Could you check a few things on this model? Use its own coordinates, in mm. A direction names the side the tool comes from. Coordinates: 2 decimals unless noted, no trailing zeros. Write each loop counter-clockwise with the first axis right and the second up, starting at its lowest first coordinate (ties: lowest second). Pieces come first, ordered by that corner, then holes. Notation, with made-up numbers: M -28.75,87.25 L 11.25,87.25 A24 ccw 11.25,116.25 Z; hole C 53.25,59 d11. An arc over 180 degrees is marked long. Write item = value, one per line.
```python
from build123d import *

# Parameters (mm, degrees)
SKETCH1_R                 = 4
BOSS_EXTRUDE1_DEPTH       = 5
SKETCH2_R                 = 6
SKETCH2_R_2               = 4
BOSS_EXTRUDE2_DEPTH       = 20
FILLET1_R                 = 5
FILLET2_R                 = 0.5
SKETCH3_R                 = 2
CUT_EXTRUDE3_DEPTH        = 5
CUT_EXTRUDE8_REACH        = 27
SKETCH10_R                = 2.5
CUT_EXTRUDE10_REACH       = 27
SKETCH13_R                = 1.5
CUT_EXTRUDE11_REACH       = 27
SKETCH14_R                = 2.1
LPATTERN1_COUNT           = 2
LPATTERN1_PITCH           = 12.2
F_4_0MM_DOWEL_HOLE1_D     = 4
F_4_0MM_DOWEL_HOLE1_DEPTH = 5
SKETCH20_R                = 2.5
CUT_EXTRUDE12_DEPTH       = 10


with BuildPart() as part:
    # Sketch1 → Boss-Extrude1 (new body)
    with BuildSketch(Plane(origin=(0, 0, 0), x_dir=(1, 0, 0), z_dir=(0, 1, 0))):
        with BuildLine():
            Line((-96.298040918, -19.992383229), (80.454801266, -20))
            ThreePointArc((80.454801266, -20), (83.283228391, -18.828427125), (84.454801266, -16))
            Line((84.454801266, -16), (84.454801266, 16.211278603))
            ThreePointArc((84.454801266, 16.211278603), (84.318504571, 17.246554783), (83.918902881, 18.211278603))
            Line((83.918902881, 18.211278603), (39.421480269, 95.283075373))
            ThreePointArc((39.421480269, 95.283075373), (37.957378654, 96.747176988), (35.957378654, 97.283075373))
            Line((35.957378654, 97.283075373), (-51.799862263, 97.283075373))
            ThreePointArc((-51.799862263, 97.283075373), (-53.799862263, 96.747176988), (-55.263963878, 95.283075373))
            Line((-55.263963878, 95.283075373), (-99.76138649, 18.211278603))
            ThreePointArc((-99.76138649, 18.211278603), (-100.16098818, 17.246554783), (-100.297284875, 16.211278603))
            Line((-100.297284875, 16.211278603), (-100.297284875, -15.992383301))
            ThreePointArc((-100.297284875, -15.992383301), (-99.125979289, -18.820543111), (-96.298040918, -19.992383229))
        make_face()
        with Locations((15, 0)):
            Circle(SKETCH1_R, mode=Mode.SUBTRACT)
        with BuildLine():
            Line((-27, 2.5), (-83, 2.5))
            ThreePointArc((-83, 2.5), (-84.414213562, 1.914213562), (-85, 0.5))
            Line((-85, 0.5), (-85, -0.5))
            ThreePointArc((-85, -0.5), (-84.414213562, -1.914213562), (-83, -2.5))
            Line((-83, -2.5), (-27, -2.5))
            ThreePointArc((-27, -2.5), (-25.585786438, -1.914213562), (-25, -0.5))
            Line((-25, -0.5), (-25, 0.5))
            ThreePointArc((-25, 0.5), (-25.585786438, 1.914213562), (-27, 2.5))
        make_face(mode=Mode.SUBTRACT)
    extrude(amount=BOSS_EXTRUDE1_DEPTH)

    # Sketch2 → Boss-Extrude2 (add)
    with BuildSketch(Plane(origin=(0, 5, 0), x_dir=(1, 0, 0), z_dir=(0, 1, 0))):
        with Locations((15, 0)):
            Circle(SKETCH2_R)
        with Locations((15, 0)):
            Circle(SKETCH2_R_2, mode=Mode.SUBTRACT)
    extrude(amount=BOSS_EXTRUDE2_DEPTH)

    # Fillet1
    fillet1_edges = [part.edges().sort_by_distance(p)[0] for p in [
        (9, 5, 0),
    ]]
    fillet(fillet1_edges, radius=FILLET1_R)

    # Fillet2
    fillet2_edges = [part.edges().sort_by_distance(p)[0] for p in [
        (9, 25, 0),
    ]]
    fillet(fillet2_edges, radius=FILLET2_R)

    # Sketch3 → Cut-Extrude3 (cut)
    with BuildSketch(Plane(origin=(0, 5, 0), x_dir=(1, 0, 0), z_dir=(0, 1, 0))):
        with Locations((-30, 15)):
            Circle(SKETCH3_R)
        with Locations((-30, -15)):
            Circle(SKETCH3_R)
    cut_extrude3 = extrude(amount=-CUT_EXTRUDE3_DEPTH, mode=Mode.SUBTRACT)

    # Mirror1: Cut-Extrude3 across plane
    add(cut_extrude3.mirror(Plane(origin=(0, 0, 0), x_dir=(0, 0, 1), z_dir=(1, 0, 0))), mode=Mode.SUBTRACT)

    # Sketch10 → Cut-Extrude8 (cut, up to next)
    with BuildSketch(Plane.XZ, mode=Mode.PRIVATE) as cut_extrude8_sk1:
        with Locations((-18, -90)):
            Circle(SKETCH10_R)
    cut_extrude8_tool1 = extrude(cut_extrude8_sk1.sketch, amount=-CUT_EXTRUDE8_REACH, mode=Mode.PRIVATE) & part.part
    add(cut_extrude8_tool1.solids().sort_by_distance((-18, 0, -90))[0], mode=Mode.SUBTRACT)
    # Sketch10 → Cut-Extrude8 (cut, up to next)
    with BuildSketch(Plane.XZ, mode=Mode.PRIVATE) as cut_extrude8_sk2:
        with Locations((2, -90)):
            Circle(SKETCH10_R)
    cut_extrude8_tool2 = extrude(cut_extrude8_sk2.sketch, amount=-CUT_EXTRUDE8_REACH, mode=Mode.PRIVATE) & part.part
    add(cut_extrude8_tool2.solids().sort_by_distance((2, 0, -90))[0], mode=Mode.SUBTRACT)

    # Sketch13 → Cut-Extrude10 (cut, up to next)
    with BuildSketch(Plane(origin=(0, 0, 0), x_dir=(-1, 0, 0), z_dir=(0, -1, 0)), mode=Mode.PRIVATE) as cut_extrude10_sk1:
        with Locations((95.647284875, -4.992383229)):
            Circle(SKETCH13_R)
    cut_extrude10_tool1 = extrude(cut_extrude10_sk1.sketch, amount=-CUT_EXTRUDE10_REACH, mode=Mode.PRIVATE) & part.part
    add(cut_extrude10_tool1.solids().sort_by_distance((-95.647285, 0, 4.992383))[0], mode=Mode.SUBTRACT)
    # Sketch13 → Cut-Extrude10 (cut, up to next)
    with BuildSketch(Plane(origin=(0, 0, 0), x_dir=(-1, 0, 0), z_dir=(0, -1, 0)), mode=Mode.PRIVATE) as cut_extrude10_sk2:
        with Locations((95.647284875, 5.007616771)):
            Circle(SKETCH13_R)
    cut_extrude10_tool2 = extrude(cut_extrude10_sk2.sketch, amount=-CUT_EXTRUDE10_REACH, mode=Mode.PRIVATE) & part.part
    add(cut_extrude10_tool2.solids().sort_by_distance((-95.647285, 0, -5.007617))[0], mode=Mode.SUBTRACT)

    # Sketch14 → Cut-Extrude11 (cut, up to next)
    with BuildSketch(Plane.XZ, mode=Mode.PRIVATE) as cut_extrude11_sk1:
        with Locations((-65.047284875, 4.992383229)):
            Circle(SKETCH14_R)
    cut_extrude11_tool1 = extrude(cut_extrude11_sk1.sketch, amount=-CUT_EXTRUDE11_REACH, mode=Mode.PRIVATE) & part.part
    add(cut_extrude11_tool1.solids().sort_by_distance((-65.047285, 0, 4.992383))[0], mode=Mode.SUBTRACT)
    # Sketch14 → Cut-Extrude11 (cut, up to next)
    with BuildSketch(Plane.XZ, mode=Mode.PRIVATE) as cut_extrude11_sk2:
        with Locations((-65.047284875, -5.007616771)):
            Circle(SKETCH14_R)
    cut_extrude11_tool2 = extrude(cut_extrude11_sk2.sketch, amount=-CUT_EXTRUDE11_REACH, mode=Mode.PRIVATE) & part.part
    add(cut_extrude11_tool2.solids().sort_by_distance((-65.047285, 0, -5.007617))[0], mode=Mode.SUBTRACT)

    # Sketch16 → Ø5.0mm Dowel Hole1 (revolve, cut)
    with BuildSketch(Plane(origin=(-7.921241804, 0, -62.283075373), x_dir=(0, 0, -1), z_dir=(1, 0, 0))):
        Polygon((0, 0), (0, 9.002151548), (2.5, 7.5), (2.5, 0), align=None)
    f_5_0mm_dowel_hole1 = revolve(axis=Axis((-7.921241804, -6.35, -62.283075373), (0, 1, 0)), mode=Mode.SUBTRACT)

    # LPattern1: Ø5.0mm Dowel Hole1 ×2
    with Locations(*[(i * LPATTERN1_PITCH, 0, 0) for i in range(1, LPATTERN1_COUNT)]):
        add(f_5_0mm_dowel_hole1, mode=Mode.SUBTRACT)

    # CirPattern1 copy 1 sketch → CirPattern1 copy 1 (revolve, cut)
    with BuildSketch(Plane(origin=(-7.921241804, 0, -74.483075373), x_dir=(-1, 0, 0), z_dir=(0, 0, -1))):
        Polygon((0, 0), (0, 9.002151548), (2.5, 7.5), (2.5, 0), align=None)
    revolve(axis=Axis((-7.921241804, -6.35, -74.483075373), (0, 1, 0)), mode=Mode.SUBTRACT)

    # CirPattern1 copy 2 sketch → CirPattern1 copy 2 (revolve, cut)
    with BuildSketch(Plane(origin=(-20.121241804, 0, -62.283075373), x_dir=(0, 0, 1), z_dir=(-1, 0, 0))):
        Polygon((0, 0), (0, 9.002151548), (2.5, 7.5), (2.5, 0), align=None)
    revolve(axis=Axis((-20.121241804, -6.35, -62.283075373), (0, 1, 0)), mode=Mode.SUBTRACT)

    # CirPattern1 copy 3 sketch → CirPattern1 copy 3 (revolve, cut)
    with BuildSketch(Plane(origin=(-7.921241804, 0, -50.083075373), x_dir=(1, 0, 0), z_dir=(0, 0, 1))):
        Polygon((0, 0), (0, 9.002151548), (2.5, 7.5), (2.5, 0), align=None)
    revolve(axis=Axis((-7.921241804, -6.35, -50.083075373), (0, 1, 0)), mode=Mode.SUBTRACT)

    # CirPattern1 copy 4 sketch → CirPattern1 copy 4 (revolve, cut)
    with BuildSketch(Plane(origin=(-7.921241804, 0, -62.283075373), x_dir=(-1, 0, 0), z_dir=(0, 0, -1))):
        Polygon((0, 0), (0, 9.002151548), (2.5, 7.5), (2.5, 0), align=None)
    revolve(axis=Axis((-7.921241804, -6.35, -62.283075373), (0, 1, 0)), mode=Mode.SUBTRACT)

    # CirPattern1 copy 5 sketch → CirPattern1 copy 5 (revolve, cut)
    with BuildSketch(Plane(origin=(-7.921241804, 0, -62.283075373), x_dir=(0, 0, 1), z_dir=(-1, 0, 0))):
        Polygon((0, 0), (0, 9.002151548), (2.5, 7.5), (2.5, 0), align=None)
    revolve(axis=Axis((-7.921241804, -6.35, -62.283075373), (0, 1, 0)), mode=Mode.SUBTRACT)

    # CirPattern1 copy 6 sketch → CirPattern1 copy 6 (revolve, cut)
    with BuildSketch(Plane(origin=(-7.921241804, 0, -62.283075373), x_dir=(1, 0, 0), z_dir=(0, 0, 1))):
        Polygon((0, 0), (0, 9.002151548), (2.5, 7.5), (2.5, 0), align=None)
    revolve(axis=Axis((-7.921241804, -6.35, -62.283075373), (0, 1, 0)), mode=Mode.SUBTRACT)

    # Ø4.0mm Dowel Hole1
    with Locations(Plane(origin=(0, 5, 0), x_dir=(1, 0, 0), z_dir=(0, 1, 0))):
        with Locations((-7.922284875, -14.996191581)):
            Hole(F_4_0MM_DOWEL_HOLE1_D / 2, depth=F_4_0MM_DOWEL_HOLE1_DEPTH)

    # Sketch20 → Cut-Extrude12 (cut)
    with BuildSketch(Plane(origin=(0, 5, 0), x_dir=(1, 0, 0), z_dir=(0, 1, 0))):
        with Locations((75, -15)):
            Circle(SKETCH20_R)
    extrude(amount=-CUT_EXTRUDE12_DEPTH, mode=Mode.SUBTRACT)


solid = part.part
```
Item 1: If we mould it in two halves opening along X, with no side actions, what happens to faces 3 (the face through (-7, 2, -97.283)), 4 (the face through (28.092, 2.535, -15.601)), 5 (the face through (-77.2, 2.46, -57.29))? For each: pulls with the +X half, pulls with the -X half, needs draft (parallel to the pull), parting line crosses it, or undercut.
Numbers:
face_3 = needs draft
face_4 = undercut
face_5 = pulls with the -X half
Item 2: I'm going to push flat-ended pins straight in: P1, Ø4, axis at x = 58, z = -23.5, coming from the -Y side; P2, Ø2, axis at x = 47.5, z = -7.5, coming from the +Y side; P3, Ø3, axis at y = 4.5, z = -82.5, coming from the -X side; P4, Ø6, axis at x = 9.5, y = 15.5, coming from the -Z side. Where does each tip first touch, or does it pass through?
Numbers:
P1 = 0
P2 = 5
P3 = -63.51
P4 = -5.45
Item 3: Imagine slicing it at A-A (x = -40). Write out the boundary of the cut face in (y, z).
Numbers:
outline = M 0,-97.28 L 5,-97.28 L 5,-2.5 L 0,-2.5 Z; M 0,2.5 L 5,2.5 L 5,19.99 L 0,19.99 Z
Item 4: If I drill on line 1 along X through (y, z) = (3.4, 15); line 2 along X through (y, z) = (1.75, -15); line 3 along Z through (x, y) = (-34, 2.25), over which ranges is the centre line in solid material (lowest first)?
Numbers:
line_1 = -100.3 to -32, -28 to -9.92, -5.92 to 28, 32 to 72.5, 77.5 to 84.45
line_2 = -100.3 to -32, -28 to 28, 32 to 84.45
line_3 = -97.28 to -2.5, 2.5 to 20
Item 5: Imagine slicing it at B-B (z = -90). Write out the boundary of the cut face in (x, y), and give its area (3 significant figures).
Numbers:
outline = M -58.31,0 L -20.5,0 L -20.5,5 L -58.31,5 Z; M -15.5,0 L -0.5,0 L -0.5,5 L -15.5,5 Z; M 4.5,0 L 42.47,0 L 42.47,5 L 4.5,5 Z
area = 454 mm²
Item 6: Imagine slicing it at C-C (y = 22). Write out the boundary of the cut face in (x, z), and give its area (3 significant figures).
Numbers:
outline = C 15,0 d12; hole C 15,0 d8
area = 62.8 mm²
Item 7: Imagine slicing it at D-D (x = 15). Write out the boundary of the cut face in (y, z).
Numbers:
outline = M 0,-97.28 L 5,-97.28 L 5,-11 A5 cw 10,-6 L 24.5,-6 A0.5 ccw 25,-5.5 L 25,-4 L 0,-4 Z; M 0,4 L 25,4 L 25,5.5 A0.5 ccw 24.5,6 L 10,6 A5 cw 5,11 L 5,20 L 0,20 Z
Item 8: For faces 1 (the face through (-55, 2, 2.5)), 2 (the face through (61.98, 2.46, -56.21)), which set-ups out of +Z, -Z, +X, -X, +Y, -Y let a thin tool reach every point of the face, with its end or its side?
Numbers:
face_1 = +Y, -Y
face_2 = -Z, +X, +Y, -Y
